from build123d import *

# Parameters (mm, degrees)
SKETCH1_R           = 9.9568
BOSS_EXTRUDE1_DEPTH = 1.2192
SKETCH2_R           = 3.5179
SKETCH2_R_2         = 2.5019
BOSS_EXTRUDE2_DEPTH = 2.9464
SKETCH3_R           = 1.0795
SKETCH3_R_2         = 0.6223
CUT_EXTRUDE1_DEPTH  = 15.386000328


with BuildPart() as part:
    # Sketch1 → Boss-Extrude1 (new body)
    with BuildSketch(Plane(origin=(0, 0, 0), x_dir=(1, 0, 0), z_dir=(0, 1, 0))):
        with Locations(Location((0, 0, 0), (0, 0, 270))):
            Circle(SKETCH1_R)
    extrude(amount=BOSS_EXTRUDE1_DEPTH)

    # Sketch2 → Boss-Extrude2 (add)
    with BuildSketch(Plane(origin=(0, 1.2192, 0), x_dir=(1, 0, 0), z_dir=(0, 1, 0))):
        with Locations(Location((0, 0, 0), (0, 0, 270))):
            Circle(SKETCH2_R)
        with Locations(Location((0, 0, 0), (0, 0, 270))):
            Circle(SKETCH2_R_2, mode=Mode.SUBTRACT)
    extrude(amount=BOSS_EXTRUDE2_DEPTH)

    # Sketch3 → Cut-Extrude1 (cut, through all)
    with BuildSketch(Plane(origin=(0, 1.2192, 0), x_dir=(1, 0, 0), z_dir=(0, 1, 0))):
        with Locations(Location((0, 0, 0), (0, 0, 270))):
            Circle(SKETCH3_R)
        with Locations(Location((-4.5212, 0, 0), (0, 0, 270))):
            Circle(SKETCH3_R_2)
        with Locations(Location((-6.54685, 0, 0), (0, 0, 270))):
            Circle(SKETCH3_R_2)
        with Locations(Location((-8.5725, 0, 0), (0, 0, 270))):
            Circle(SKETCH3_R_2)
        with Locations(Location((8.5725, 0, 0), (0, 0, 90))):
            Circle(SKETCH3_R_2)
        with Locations(Location((6.54685, 0, 0), (0, 0, 90))):
            Circle(SKETCH3_R_2)
        with Locations(Location((4.5212, 0, 0), (0, 0, 90))):
            Circle(SKETCH3_R_2)
        with Locations(Location((0, 4.5212, 0), (0, 0, 270))):
            Circle(SKETCH3_R_2)
        with Locations(Location((0, 6.54685, 0), (0, 0, 270))):
            Circle(SKETCH3_R_2)
        with Locations(Location((0, 8.5725, 0), (0, 0, 270))):
            Circle(SKETCH3_R_2)
        with Locations(Location((0, -4.5212, 0), (0, 0, 90))):
            Circle(SKETCH3_R_2)
        with Locations(Location((0, -6.54685, 0), (0, 0, 90))):
            Circle(SKETCH3_R_2)
        with Locations(Location((0, -8.5725, 0), (0, 0, 90))):
            Circle(SKETCH3_R_2)
    extrude(amount=-CUT_EXTRUDE1_DEPTH, mode=Mode.SUBTRACT)


solid = part.part
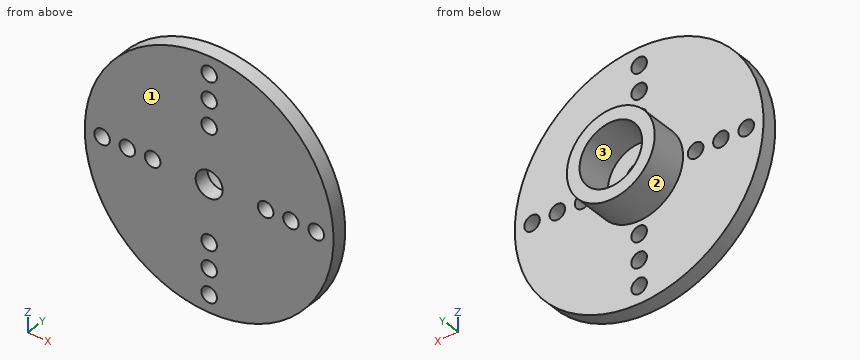
Geometry check sheet. Reference: the model listing, model coordinates, mm. Face numbers are marked on the shaded views. Round coordinates to 2 decimals unless told otherwise and drop trailing zeros. Write each loop counter-clockwise with the first axis right and the second up, starting at its lowest first coordinate (ties: lowest second). Pieces come first, ordered by that corner, then holes.
Item 1: Section check B-B (y = 2.45). Record the boundary of the cut face in (x, z).
Determined:
outline: circle Ø7.04 at (0, 0); hole circle Ø5 at (0, 0)
Item 2: Section check C-C (x = 0). Give the number of separate pieces and of enclosed holes in the cut face, plus the area to 3 significant figures.
Determined:
separate pieces: 8
enclosed holes: 0
area: 18.5 mm2
Item 3: Section check A-A (z = 6.75). Record the boundary of the cut face in (x, y), plus the area to 3 significant figures.
Determined:
outline: (-7.32, 0) - (-0.59, 0) - (-0.59, 1.22) - (-7.32, 1.22) - close; (0.59, 0) - (7.32, 0) - (7.32, 1.22) - (0.59, 1.22) - close
area: 16.4 mm2
Item 4: Mould release check, pull along X, two halves, no side actions. Record for the marked faces 1, 2 and 3: +X half, -X half, draft (parallel to the pull), parting line (faces both ways), or undercut.
Determined:
face 1: draft
face 2: parting line
face 3: undercut
Item 5: Go/stop test with flat-tipped pins: pin 1 Ø2 at (x, z) = (-8.57, 0) entering from +Y; pin 2 Ø2 at (x, z) = (0, 6.55) entering from -Y; pin 3 Ø2 at (x, y) = (1, 2.5) entering from -Z; pin 4 Ø1.5 at (y, z) = (3, -4) entering from +X. Record where each tip stops, or that it passes through.
Determined:
pin 1: stops at y = 1.22
pin 2: stops at y = 0
pin 3: stops at z = -3.52
pin 4: stops at x = 1.35
Item 6: Material ranges on line 1 along Y through (x, z) = (3, -3.75); line 2 along Z through (x, y) = (-1, 3.7); line 3 along X through (y, z) = (0.3, -9), recorded low to high.
Determined:
line 1: y = 0 to 1.22
line 2: z = -3.37 to -2.29, 2.29 to 3.37
line 3: x = -4.26 to -0.45, 0.45 to 4.26
